```python
from build123d import *

# Parameters (mm, degrees)
EXTRUDE_1_DEPTH = 50
SKETCH_2_W      = 20
SKETCH_2_H      = 10
SKETCH_2_R      = 1.6
EXTRUDE_2_DEPTH = 3


with BuildPart() as part:
    # Sketch 1 → Extrude 1 (new body)
    with BuildSketch(Plane.XY):
        Polygon((-151.179701436, 97.04447756), (98.820298564, 97.04447756), (98.820298564, 95.04447756), (96.820298564, 95.04447756), (-149.179701436, 95.04447756), (-149.179701436, -46.95552244), (96.820298564, -46.95552244), (98.820298564, -46.95552244), (98.820298564, -48.95552244), (-151.179701436, -48.95552244), align=None)
    extrude(amount=EXTRUDE_1_DEPTH)

    # Sketch 2 → Extrude 2 (add)
    # profile 1 of 4: a face of its own
    with BuildSketch(Plane.XY):
        with Locations((-141.179701436, -43.95552244)):
            Rectangle(SKETCH_2_W, SKETCH_2_H)
        with Locations((-146.179701436, -43.95552244)):
            Circle(SKETCH_2_R, mode=Mode.SUBTRACT)
        with Locations((-136.179701436, -43.95552244)):
            Circle(SKETCH_2_R, mode=Mode.SUBTRACT)
    # profile 2 of 4: a face of its own
    with BuildSketch(Plane.XY):
        with Locations((88.820298564, -43.95552244)):
            Rectangle(SKETCH_2_W, SKETCH_2_H)
        with Locations(Location((83.820298564, -43.95552244, 0), (0, 0, 180))):
            Circle(SKETCH_2_R, mode=Mode.SUBTRACT)
        with Locations(Location((93.820298564, -43.95552244, 0), (0, 0, 180))):
            Circle(SKETCH_2_R, mode=Mode.SUBTRACT)
    # profile 3 of 4: a face of its own
    with BuildSketch(Plane.XY):
        with Locations((88.820298564, 92.04447756)):
            Rectangle(SKETCH_2_W, SKETCH_2_H)
        with Locations((93.820298564, 92.04447756)):
            Circle(SKETCH_2_R, mode=Mode.SUBTRACT)
        with Locations((83.820298564, 92.04447756)):
            Circle(SKETCH_2_R, mode=Mode.SUBTRACT)
    # profile 4 of 4: a face of its own
    with BuildSketch(Plane.XY):
        with Locations((-141.179701436, 92.04447756)):
            Rectangle(SKETCH_2_W, SKETCH_2_H)
        with Locations(Location((-136.179701436, 92.04447756, 0), (0, 0, 180))):
            Circle(SKETCH_2_R, mode=Mode.SUBTRACT)
        with Locations(Location((-146.179701436, 92.04447756, 0), (0, 0, 180))):
            Circle(SKETCH_2_R, mode=Mode.SUBTRACT)
    extrude(amount=EXTRUDE_2_DEPTH)


solid = part.part
```
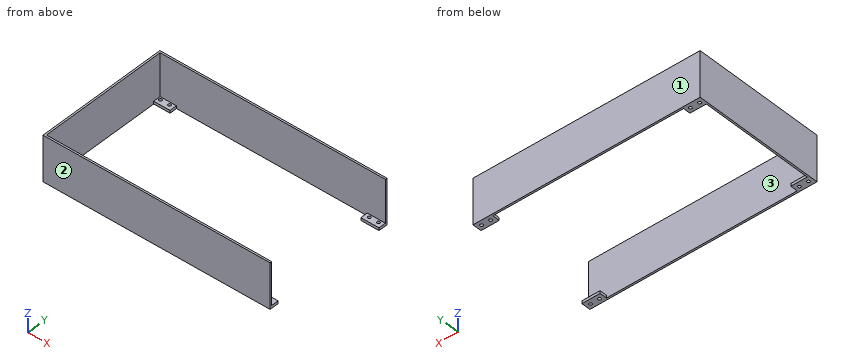
Input: part model. Units: mm. Frame: model coordinates. Face numbers are marked on the shaded views. Coordinates: 2 decimals unless noted, no trailing zeros. Order: outer loops, then holes, each group sorted by start corner. A loop starts at its lowest first (then second) coordinate and runs counter-clockwise, first axis right, second up. Notation, with made-up numbers: (74, -8) - (109, -8) arc R29 ccw to (109, 30) - close; hole circle Ø2 at (63.5, 82.5). An arc over 180 degrees is marked (long way). Return JSON: item names as keys, results as strings.
Q1. Cut plane C-C (y = 82). Return loops of the section in (x, z).
The answers:
{"outline": "(-151.18, 0) - (-149.18, 0) - (-149.18, 50) - (-151.18, 50) - close"}
Q2. First-contact query: pin 1 (10 mm diameter, centred on y = 46.5, z = 14.5, fed in from +X); pin 2 (2.5 mm diameter, centred on x = -139, y = 89.5, fed in from +Z). Flat tips, straight axial feed; report the tip coordinate or a pass-through.
The answers:
{"pin 1": "stops at x = -149.18", "pin 2": "stops at z = 3"}
Q3. Cut plane B-B (z = 11). Return loops of the section in (x, y).
The answers:
{"outline": "(-151.18, -48.96) - (98.82, -48.96) - (98.82, -46.96) - (-149.18, -46.96) - (-149.18, 95.04) - (98.82, 95.04) - (98.82, 97.04) - (-151.18, 97.04) - close"}
Q4. Ray query, probe 1 along Y at (x, z) = (-49, 17); probe 2 along X at (y, z) = (82, 23.5). Return the intervals inside material, ascending.
The answers:
{"probe 1": "y = -48.96 to -46.96, 95.04 to 97.04", "probe 2": "x = -151.18 to -149.18"}
Q5. Cut plane A-A (x = 29). Return loops of the section in (y, z), then the cut area to 3 significant figures.
The answers:
{"outline": "(-48.96, 0) - (-46.96, 0) - (-46.96, 50) - (-48.96, 50) - close; (95.04, 0) - (97.04, 0) - (97.04, 50) - (95.04, 50) - close", "area": "200 mm2"}
Q6. Draft query along Y for the marked faces 1, 2 and 3. Return one class per face: +Y half, -Y half, draft (parallel to the pull), parting line (faces both ways), or undercut.
The answers:
{"face 1": "+Y half", "face 2": "-Y half", "face 3": "undercut"}
